Verification items for the finished model (mm, model axes). A direction names the side the tool comes from. Coordinates: 2 decimals unless noted, no trailing zeros. Write each loop counter-clockwise with the first axis right and the second up, starting at its lowest first coordinate (ties: lowest second). Pieces come first, ordered by that corner, then holes. Notation, with made-up numbers: M 66,17.5 L 86,17.5 A17 cw 86,39.5 Z; hole C -23,18 d6. An arc over 180 degrees is marked long. One line per item, written item: value.
```python
from build123d import *

# Parameters (mm, degrees)
F1_DEPTH = 15
F4_D     = 3.5
F4_DEPTH = 14.5
F5_R     = 3


with BuildPart() as f1:
    # F0 (on Front) → F1 (new body)
    with BuildSketch(Plane.XZ):
        with BuildLine():
            ThreePointArc((-21, -35.271837), (-35.6872, -20.28611), (-41.05, 0))
            Line((-41.05, 0), (-60.83, 0))
            Line((-60.83, 0), (-60.83, -4.5))
            Line((-60.83, -4.5), (-48.83, -4.5))
            Line((-48.83, -4.5), (-44.731143, -10.942))
            ThreePointArc((-44.731143, -10.942), (-37.395384, -26.873551), (-24.634821, -38.906659))
            Line((-24.634821, -38.906659), (-21, -35.271837))
        make_face()
        with BuildLine():
            ThreePointArc((41.05, 0), (35.6872, -20.28611), (21, -35.271837))
            Line((21, -35.271837), (24.634821, -38.906659))
            ThreePointArc((24.634821, -38.906659), (37.395384, -26.873551), (44.731143, -10.942))
            Line((44.731143, -10.942), (48.83, -4.5))
            Line((48.83, -4.5), (60.83, -4.5))
            Line((60.83, -4.5), (60.83, 0))
            Line((60.83, 0), (41.05, 0))
        make_face()
        with BuildLine():
            ThreePointArc((11.744722, -44.527115), (0, -46.05), (-11.744722, -44.527115))
            Line((-11.744722, -44.527115), (-15.379543, -48.161937))
            ThreePointArc((-15.379543, -48.161937), (0, -50.557912), (15.379543, -48.161937))
            Line((15.379543, -48.161937), (11.744722, -44.527115))
        make_face()
        Polygon((-11.744722, -44.527115), (-21, -35.271837), (-24.634821, -38.906659), (-15.379543, -48.161937), align=None)
        Polygon((24.634821, -38.906659), (21, -35.271837), (11.744722, -44.527115), (15.379543, -48.161937), align=None)
    extrude(amount=F1_DEPTH)

    # F4
    with Locations(Plane(origin=(0, 0, -4.5), x_dir=(1, 0, 0), z_dir=(0, 0, -1))):
        with Locations((-54.83, 7.5), (54.83, 7.5)):
            Hole(F4_D / 2, depth=F4_DEPTH)

    # F5
    f5_edges = [f1.edges().sort_by_distance(p)[0] for p in [
        (-60.83, 0, -2.25),
        (-54.83, 0, -4.5),
        (-60.83, -7.5, -4.5),
        (-60.83, -15, -2.25),
        (-54.83, -15, -4.5),
        (-46.780571, -15, -7.721),
        (-46.780571, 0, -7.721),
        (-20.007182, 0, -43.534298),
        (-37.395384, 0, -26.873551),
        (0, 0, -50.557912),
        (20.007182, 0, -43.534298),
        (37.395384, 0, -26.873551),
        (46.780571, 0, -7.721),
        (54.83, 0, -4.5),
        (60.83, -7.5, -4.5),
        (60.83, -15, -2.25),
        (54.83, -15, -4.5),
        (46.780571, -15, -7.721),
        (-20.007182, -15, -43.534298),
        (0, -15, -50.557912),
        (20.007182, -15, -43.534298),
        (37.395384, -15, -26.873551),
        (-37.395384, -15, -26.873551),
        (60.83, 0, -2.25),
    ]]
    fillet(f5_edges, radius=F5_R)


solid = f1.part
```
Item 1: Scan lines: line 1 (X direction, y = -7.5, z = -1); line 2 (X direction, y = -7.5, z = -3.2); line 3 (Y direction, x = -54.83, z = -0.95). Record each from-to range of solid material in increasing order.
The answers:
line 1: x = -60.83 to -56.58, -53.08 to -41.04, 41.04 to 53.08, 56.58 to 60.83
line 2: x = -60.3 to -56.58, -53.08 to -40.93, 40.93 to 53.08, 56.58 to 60.3
line 3: y = -15 to -9.25, -5.75 to 0
Item 2: Cross-section at B-B, the plane y = -7.5. Enter the section's corners in (x, z), and give its area (3 significant figures).
The answers:
outline: M -60.83,-1.5 A3 ccw -57.83,-4.5 L -56.58,-4.5 L -56.58,0 L -60.83,0 Z; M -53.08,-4.5 L -48.83,-4.5 L -44.73,-10.94 A46.05 ccw -24.63,-38.91 L -15.38,-48.16 A50.56 ccw 15.38,-48.16 L 24.63,-38.91 A46.05 ccw 44.73,-10.94 L 48.83,-4.5 L 53.08,-4.5 L 53.08,0 L 41.05,0 A41.05 cw 21,-35.27 L 11.74,-44.53 A46.05 cw -11.74,-44.53 L -21,-35.27 A41.05 cw -41.05,0 L -53.08,0 Z; M 56.58,-4.5 L 57.83,-4.5 A3 ccw 60.83,-1.5 L 60.83,0 L 56.58,0 Z
area: 819 mm²
Item 3: Access from +Z, -Z, +X, -X, +Y, -Y to the whole of each face (thin tool, end or side, straight path). Record for faces 5 (the face through (-52, -7, -4.5)), 6 (the face through (16.44, -7.4, -39.83)), 7 (the face through (-51, -7, 0)).
The answers:
face 5: -Z, -X, +Y, -Y
face 6: +Z, +Y, -Y
face 7: +Z, +X, -X, +Y, -Y
Item 4: Cross-section at C-C, the plane y = -1.25. Enter the section's corners in (x, z).
The answers:
outline: M -60.27,-1.5 A2.44 ccw -57.83,-3.94 L -48.52,-3.94 L -44.21,-10.72 A45.49 ccw -24.28,-38.46 L -15.08,-47.67 A49.99 ccw 15.08,-47.67 L 24.28,-38.46 A45.49 ccw 44.21,-10.72 L 48.52,-3.94 L 57.83,-3.94 A2.44 ccw 60.27,-1.5 L 60.27,0 L 41.05,0 A41.05 cw 21,-35.27 L 11.74,-44.53 A46.05 cw -11.74,-44.53 L -21,-35.27 A41.05 cw -41.05,0 L -60.27,0 Z
Item 5: Draft check along X on faces 1 (the face through (-46.29, -14.145, -6.812)), 2 (the face through (53.213, -6.83, -2.218)), 3 (the face through (-52.43, -14.14, -3.6)), 4 (the face through (59.93, -7.56, -3.64)). Enter one of: released by +X, released by -X, zero draft, split by the parting line, or undercut.
The answers:
face 1: released by -X
face 2: undercut
face 3: zero draft
face 4: released by +X
Item 6: Cross-section at A-A, the plane x = 54.83. Enter the section's corners in (y, z), and give its area (3 significant figures).
The answers:
outline: M -15,-1.5 A3 ccw -12,-4.5 L -9.25,-4.5 L -9.25,0 L -15,0 Z; M -5.75,-4.5 L -3,-4.5 A3 ccw 0,-1.5 L 0,0 L -5.75,0 Z
area: 47.9 mm²
Item 7: Go/stop test with flat-tipped pins: P1, Ø4.5, axis at x = 52, y = -6, coming from the -Z side; P2, Ø3, axis at x = 17, y = -2, coming from the +Z side; P3, Ø3, axis at x = 54.83, y = -7.5, coming from the -Z side; P4, Ø1.5, axis at y = -12, z = -31, coming from the +X side. Record where each tip stops, or that it passes through.
The answers:
P1: stops at z = -4.5
P2: stops at z = -37.77
P3: passes through
P4: stops at x = 34.72
